Geometry check sheet. Reference: the model listing, model coordinates, mm. Face numbers are marked on the shaded views. A direction names the side the tool comes from. Give positions to 0.01 mm unless a question says otherwise; leave off trailing zeros. Write each loop counter-clockwise with the first axis right and the second up, starting at its lowest first coordinate (ties: lowest second). Pieces come first, ordered by that corner, then holes. Notation, with made-up numbers: M 4,23 L 47,23 A23 cw 47,47 Z; hole C 73.5,73 d2. An arc over 180 degrees is marked long. One line per item, written item: value. Start each with the question number.
1. Cross-section at C-C on x = 18. Record the cut outline in (y, z).
2. Cross-section at A-A on z = 32.5. Record the cut outline in (x, y), then the cut area to 3 significant figures.
3. Cross-section at B-B on z = 17.5. Record the cut outline in (x, y), then the cut area to 3 significant figures.
4. Gauge pin test, flat ends, axial feed: pin 1 (1 mm diameter, centred on x = 74, y = 10.5, fed in from +Z); pin 2 (1.4 mm diameter, centred on x = 73, z = 54, fed in from +Y); pin 3 (3 mm diameter, centred on x = 82.85, y = 17.78, fed in from -Z). Record the tip position at first contact, or that the pin passes through.
5. Scan lines: line 1 (Y direction, x = 5, z = 48); line 2 (X direction, y = 15.75, z = 24); line 3 (Z direction, x = 101.5, y = 12.25). Record each from-to range of solid material in increasing order.
6. Cross-section at D-D on y = 17.78. Record the cut outline in (x, z), then the cut area to 3 significant figures.
7. Tool access check on the marked faces 1, 2 and 3. Record the directions out of +Z, -Z, +X, -X, +Y, -Y that give a thin tool (end or side, any length) a straight path to the whole face; none if there is none.
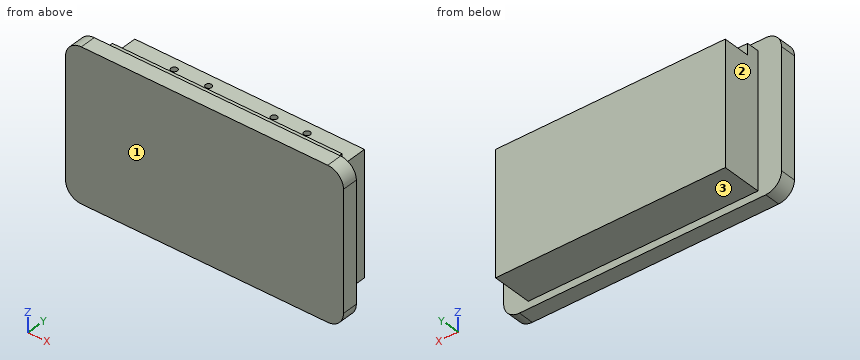
from build123d import *

# Parameters (mm, degrees)
F1_DEPTH = 6.35
F2_W     = 92.6338
F2_H     = 54.0004
F3_DEPTH = 5.08
F4_W     = 92.6338
F4_H     = 49.4792
F5_DEPTH = 11.0236
F6_R     = 1.27
F7_DEPTH = 25.4


with BuildPart() as f1:
    # F0 (on Front) → F1 (new body)
    with BuildSketch(Plane.XZ):
        with BuildLine():
            ThreePointArc((0, 6.35), (1.859872, 1.859872), (6.35, 0))
            Line((6.35, 0), (105.7148, 0))
            ThreePointArc((105.7148, 0), (110.204928, 1.859872), (112.0648, 6.35))
            Line((112.0648, 6.35), (112.0648, 54.1782))
            ThreePointArc((112.0648, 54.1782), (110.204928, 58.668328), (105.7148, 60.5282))
            Line((105.7148, 60.5282), (6.35, 60.5282))
            ThreePointArc((6.35, 60.5282), (1.859872, 58.668328), (0, 54.1782))
            Line((0, 54.1782), (0, 6.35))
        make_face()
    extrude(amount=-F1_DEPTH)

    # F2 (on face) → F3 (join)
    with BuildSketch(Plane(origin=(0, 6.35, 0), x_dir=(-1, 0, 0), z_dir=(0, 1, 0))):
        with Locations((-55.8165, 29.9212)):
            Rectangle(F2_W, F2_H)
    extrude(amount=F3_DEPTH)

    # F4 (on face) → F5 (join)
    with BuildSketch(Plane(origin=(0, 11.43, 0), x_dir=(-1, 0, 0), z_dir=(0, 1, 0))):
        with Locations((-55.8165, 27.6606)):
            Rectangle(F4_W, F4_H)
    extrude(amount=F5_DEPTH)

    # F6 (on face) → F7 (cut)
    with BuildSketch(Plane.XY.offset(52.4002)):
        with Locations((29.2608, 17.78)):
            Circle(F6_R)
        with Locations((43.1546, 17.78)):
            Circle(F6_R)
        with Locations((69.4944, 17.78)):
            Circle(F6_R)
        with Locations((82.8548, 17.78)):
            Circle(F6_R)
    extrude(amount=-F7_DEPTH, mode=Mode.SUBTRACT)


solid = f1.part
Report:
1. outline: M 0,0 L 6.35,0 L 6.35,2.92 L 22.45,2.92 L 22.45,52.4 L 11.43,52.4 L 11.43,56.92 L 6.35,56.92 L 6.35,60.53 L 0,60.53 Z
2. outline: M 0,0 L 112.06,0 L 112.06,6.35 L 102.13,6.35 L 102.13,22.45 L 9.5,22.45 L 9.5,6.35 L 0,6.35 Z; hole C 29.26,17.78 d2.54; hole C 43.15,17.78 d2.54; hole C 69.49,17.78 d2.54; hole C 82.85,17.78 d2.54
2. area: 2,180 mm^2
3. outline: M 0,0 L 112.06,0 L 112.06,6.35 L 102.13,6.35 L 102.13,22.45 L 9.5,22.45 L 9.5,6.35 L 0,6.35 Z
3. area: 2,200 mm^2
4. pin 1: stops at z = 56.92
4. pin 2: stops at y = 11.43
4. pin 3: stops at z = 2.92
5. line 1: y = 0 to 6.35
5. line 2: x = 9.5 to 102.13
5. line 3: z = 2.92 to 52.4
6. outline: M 9.5,2.92 L 102.13,2.92 L 102.13,52.4 L 84.12,52.4 L 84.12,27 L 81.58,27 L 81.58,52.4 L 70.76,52.4 L 70.76,27 L 68.22,27 L 68.22,52.4 L 44.42,52.4 L 44.42,27 L 41.88,27 L 41.88,52.4 L 30.53,52.4 L 30.53,27 L 27.99,27 L 27.99,52.4 L 9.5,52.4 Z
6. area: 4,330 mm^2
7. face 1: +Z, -Z, +X, -X, -Y
7. face 2: +Z, -Z, -X, +Y
7. face 3: -Z, +X, -X, +Y
